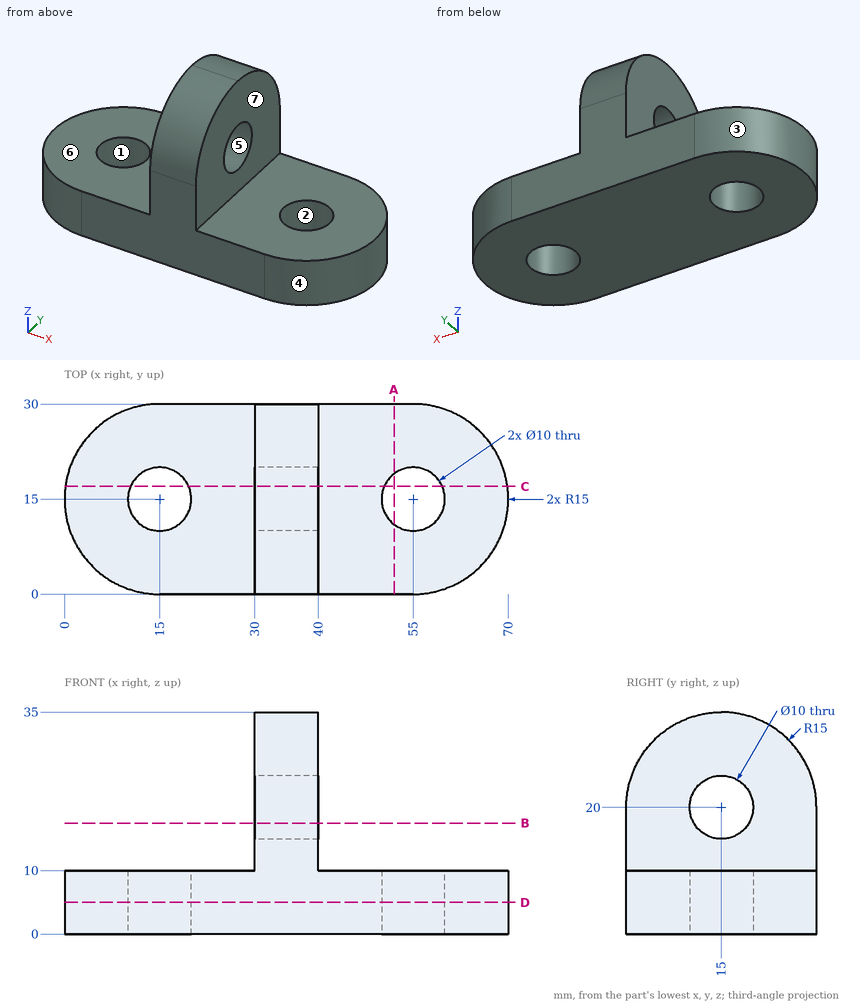
Job drawing, mm, ordinate dimensions from the low corner. One solid piece. A direction names the side the tool comes from. Give positions to 0.01 mm unless a question says otherwise; leave off trailing zeros. Loops run counter-clockwise (first coordinate to the right, second up) from the corner with the lowest first, then second, coordinate; pieces in that order, holes last. Notation, with made-up numbers: (-33.5, 84) -> (-10.5, 84) arc R20 ccw to (-10.5, 110) -> close; hole circle Ø11 at (61.25, -10). An arc over 180 degrees is marked (long way). Use a Markdown table: item, result. Add a question column.
(1) Slice it at C-C on y = 17. List the corners of the cut face in (x, z).
(2) Slice it at B-B on z = 17.5. List the corners of the cut face in (x, y).
(3) Drop flat-ended pins along their axis: pin 1 Ø12 at (y, z) = (8.5, 12.5) entering from +X; pin 2 Ø10 at (x, z) = (50.5, 19.5) entering from +Y; pin 3 Ø13 at (y, z) = (15, 20) entering from +X; pin 4 Ø3 at (y, z) = (20, 7) entering from -X. Give the stop position or say it passes through.
(4) Tool access for the marked faces 5, 6 and 7: list every direction of +Z, -Z, +X, -X, +Y, -Y with a clear straight run to the whole face (end or side of a thin tool).
(5) Mould opens along X. For the marked faces 1, 2, 3 and 4 say: +X half, -X half, draft (parallel to the pull), parting line (faces both ways), or undercut.
(6) Slice it at D-D on z = 5. List the corners of the cut face in (x, y).
(7) Wall check: line 1 along Y through (x, z) = (15, 2.75); line 2 along X through (y, z) = (4, 21); line 3 along Z through (x, y) = (16, 25). Give the ranges that are in metal, low to high.
(8) Slice it at A-A on x = 52. List the corners of the cut face in (y, z).
Filled sheet:
| question | item | result |
|---|---|---|
| 1 | outline | (0.13, 0) -> (10.42, 0) -> (10.42, 10) -> (0.13, 10) -> close; (19.58, 0) -> (50.42, 0) -> (50.42, 10) -> (40, 10) -> (40, 15.42) -> (30, 15.42) -> (30, 10) -> (19.58, 10) -> close; (30, 24.58) -> (40, 24.58) -> (40, 34.87) -> (30, 34.87) -> close; (59.58, 0) -> (69.87, 0) -> (69.87, 10) -> (59.58, 10) -> close |
| 2 | outline | (30, 0) -> (40, 0) -> (40, 10.67) -> (30, 10.67) -> close; (30, 19.33) -> (40, 19.33) -> (40, 30) -> (30, 30) -> close |
| 3 | pin 1 | x = 69.96 |
| 3 | pin 2 | through |
| 3 | pin 3 | x = 40 |
| 3 | pin 4 | x = 0.41 |
| 4 | face 5 | +X, -X |
| 4 | face 6 | +Z, -X, +Y, -Y |
| 4 | face 7 | +Z, +X, +Y, -Y |
| 5 | face 1 | undercut |
| 5 | face 2 | undercut |
| 5 | face 3 | -X half |
| 5 | face 4 | +X half |
| 6 | outline | (15, 0) -> (55, 0) arc R15 ccw to (55, 30) -> (15, 30) arc R15 ccw to start; hole circle Ø10 at (15, 15); hole circle Ø10 at (55, 15) |
| 7 | line 1 | 0 to 10, 20 to 30 |
| 7 | line 2 | 30 to 40 |
| 7 | line 3 | 0 to 10 |
| 8 | outline | (0, 0) -> (11, 0) -> (11, 10) -> (0, 10) -> close; (19, 0) -> (30, 0) -> (30, 10) -> (19, 10) -> close |
